Here's how the part is built. I have some questions about the finished solid (model axes, mm). Face numbers are marked on the shaded views. Give positions to 0.01 mm unless a question says otherwise; leave off trailing zeros. Loops run counter-clockwise (first coordinate to the right, second up) from the corner with the lowest first, then second, coordinate; pieces in that order, holes last. Notation, with made-up numbers: (17, -37.5) - (43, -37.5) arc R20 cw to (43, -18.5) - close; hole circle Ø9 at (-16, 36.25). An arc over 180 degrees is marked (long way). Use a Markdown table: item, result.
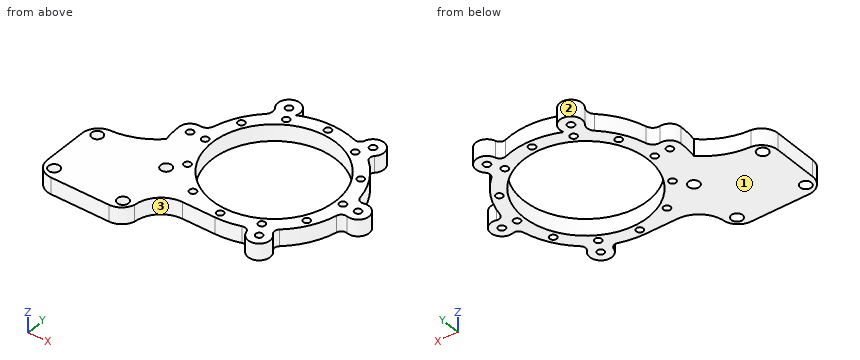
from build123d import *

# Parameters (mm, degrees)
SKETCH_2_R      = 1.25
SKETCH_2_R_2    = 22.5
SKETCH_2_R_3    = 2
EXTRUDE_1_DEPTH = 6
EXTRUDE_START   = -6
SKETCH_3_R      = 1.25
EXTRUDE_2_DEPTH = 6


with BuildPart() as part:
    # 草图2 → 凸台-拉伸1 (new body)
    with BuildSketch(Plane.XY):
        with BuildLine():
            ThreePointArc((11.071751856, 33.094337161), (3.155908846, 19.70243628), (-11.296671761, 13.946874314))
            ThreePointArc((-11.296671761, 13.946874314), (-15.015530454, 11.950947319), (-16.5, 8))
            Line((-16.5, 8), (-16.5, -8))
            ThreePointArc((-16.5, -8), (-14.742640687, -12.242640687), (-10.5, -14))
            Line((-10.5, -14), (10.5, -14))
            ThreePointArc((10.5, -14), (14.176185773, -12.741904487), (16.31070727, -9.495219388))
            ThreePointArc((16.31070727, -9.495219388), (19.407668924, -2.752662347), (26.297958971, 0))
            Line((26.297958971, 0), (37.996710384, 0))
            ThreePointArc((37.996710384, 0), (59.328544247, 44.855197033), (11.071751856, 33.094337161))
        make_face()
        with Locations((16.346075289, 15)):
            Circle(SKETCH_2_R, mode=Mode.SUBTRACT)
        with Locations((37.996710384, 2.5)):
            Circle(SKETCH_2_R, mode=Mode.SUBTRACT)
        with Locations((25.496710384, 5.849364905)):
            Circle(SKETCH_2_R, mode=Mode.SUBTRACT)
        with Locations((50.496710384, 5.849364905)):
            Circle(SKETCH_2_R, mode=Mode.SUBTRACT)
        with Locations((59.647345479, 15)):
            Circle(SKETCH_2_R, mode=Mode.SUBTRACT)
        with Locations((12.996710384, 27.5)):
            Circle(SKETCH_2_R, mode=Mode.SUBTRACT)
        with Locations((16.346075289, 40)):
            Circle(SKETCH_2_R, mode=Mode.SUBTRACT)
        with Locations((37.996710384, 27.5)):
            Circle(SKETCH_2_R_2, mode=Mode.SUBTRACT)
        with Locations((62.996710384, 27.5)):
            Circle(SKETCH_2_R, mode=Mode.SUBTRACT)
        with Locations((25.496710384, 49.150635095)):
            Circle(SKETCH_2_R, mode=Mode.SUBTRACT)
        with Locations((37.996710384, 52.5)):
            Circle(SKETCH_2_R, mode=Mode.SUBTRACT)
        with Locations((59.647345479, 40)):
            Circle(SKETCH_2_R, mode=Mode.SUBTRACT)
        with Locations((50.496710384, 49.150635095)):
            Circle(SKETCH_2_R, mode=Mode.SUBTRACT)
        with Locations((12.5, -10)):
            Circle(SKETCH_2_R_3, mode=Mode.SUBTRACT)
        with Locations((-12.5, 10)):
            Circle(SKETCH_2_R_3, mode=Mode.SUBTRACT)
        with Locations((12.5, 10)):
            Circle(SKETCH_2_R_3, mode=Mode.SUBTRACT)
        with Locations((-12.5, -10)):
            Circle(SKETCH_2_R_3, mode=Mode.SUBTRACT)
    extrude(amount=EXTRUDE_1_DEPTH)

    # 草图3 → 凸台-拉伸2 (add)
    # profile 1 of 5: a face of its own
    with BuildSketch(Plane.XY.offset(6).offset(EXTRUDE_START)):
        with BuildLine():
            ThreePointArc((67.447530056, 23.64004914), (72.496710384, 27.5), (67.447530056, 31.35995086))
            ThreePointArc((67.447530056, 31.35995086), (65.870885098, 31.588991044), (64.961839586, 32.897388914))
            ThreePointArc((64.961839586, 32.897388914), (65.496710384, 27.5), (64.961839586, 22.102611086))
            ThreePointArc((64.961839586, 22.102611086), (65.870885098, 23.411008956), (67.447530056, 23.64004914))
        make_face()
        with Locations((68.496710384, 27.5)):
            Circle(SKETCH_3_R, mode=Mode.SUBTRACT)
    # profile 2 of 5: a face of its own
    with BuildSketch(Plane.XY.offset(6).offset(EXTRUDE_START)):
        with BuildLine():
            ThreePointArc((56.064935722, 51.075182568), (55.246710384, 57.377876431), (49.379304718, 54.935133428))
            ThreePointArc((49.379304718, 54.935133428), (48.392627621, 53.684238934), (46.804999072, 53.551181363))
            ThreePointArc((46.804999072, 53.551181363), (51.746710384, 51.315698604), (56.153550899, 48.153792449))
            ThreePointArc((56.153550899, 48.153792449), (55.474967861, 49.59524789), (56.064935722, 51.075182568))
        make_face()
        with Locations((53.246710384, 53.913774815)):
            Circle(SKETCH_3_R, mode=Mode.SUBTRACT)
    # profile 3 of 5: a face of its own
    with BuildSketch(Plane.XY.offset(6).offset(EXTRUDE_START)):
        with BuildLine():
            ThreePointArc((49.379304718, 0.064866572), (55.246710384, -2.377876431), (56.064935722, 3.924817432))
            ThreePointArc((56.064935722, 3.924817432), (55.474967861, 5.40475211), (56.153550899, 6.846207551))
            ThreePointArc((56.153550899, 6.846207551), (51.746710384, 3.684301396), (46.804999072, 1.448818637))
            ThreePointArc((46.804999072, 1.448818637), (48.392627621, 1.315761066), (49.379304718, 0.064866572))
        make_face()
        with Locations((53.246710384, 1.086225185)):
            Circle(SKETCH_3_R, mode=Mode.SUBTRACT)
    # profile 4 of 5: a face of its own
    with BuildSketch(Plane.XY.offset(6).offset(EXTRUDE_START)):
        with BuildLine():
            ThreePointArc((26.477501839, 52.471140032), (22.209078662, 57.87747916), (19.535000313, 51.529468119))
            ThreePointArc((19.535000313, 51.529468119), (20.114268508, 49.473728128), (19.179054293, 47.553573727))
            ThreePointArc((19.179054293, 47.553573727), (22.630287457, 50.306206314), (26.477501839, 52.471140032))
        make_face()
        with Locations((22.746710384, 53.913774815)):
            Circle(SKETCH_3_R, mode=Mode.SUBTRACT)
    # profile 5 of 5: a face of its own
    with BuildSketch(Plane.XY.offset(6).offset(EXTRUDE_START)):
        with BuildLine():
            ThreePointArc((4.186169411, 20.637251344), (8.570590949, 26.345313518), (11.071751856, 33.094337161))
            ThreePointArc((11.071751856, 33.094337161), (11.144241114, 33.432528477), (11.220978054, 33.769781351))
            ThreePointArc((11.220978054, 33.769781351), (10.025683209, 31.99978526), (7.955726823, 31.473575708))
            ThreePointArc((7.955726823, 31.473575708), (4.835513826, 30.486307566), (3.496710384, 27.5))
            ThreePointArc((3.496710384, 27.5), (3.669507879, 24.051352697), (4.186169411, 20.637251344))
        make_face()
        with Locations((7.496710384, 27.5)):
            Circle(SKETCH_3_R, mode=Mode.SUBTRACT)
    extrude(amount=EXTRUDE_2_DEPTH)


solid = part.part
(1) Suppose I cut it at A-A on y = 35. Write out the boundary of the cut face in (x, z), plus the area to 3 significant figures.
A:
| item | result |
|---|---|
| outline | (11.54, 0) - (16.78, 0) - (16.78, 6) - (11.54, 6) - close; (59.21, 0) - (64.45, 0) - (64.45, 6) - (59.21, 6) - close |
| area | 62.9 mm2 |
(2) If I drill on line 1 (X direction, y = 16, z = 3.15); line 2 (Y direction, x = 56.5, z = 3.15); line 3 (X direction, y = -8.5, z = 3.2), over which ranges is the centre line in solid material (lowest first)?
A:
| item | result |
|---|---|
| line 1 | -2.7 to 15.6, 17.1 to 18.66, 57.34 to 58.9, 60.4 to 62.98 |
| line 2 | -1.24 to 3.41, 7.16 to 14.7, 40.3 to 47.84, 51.59 to 56.24 |
| line 3 | -16.48 to -13.82, -11.18 to 11.18, 13.82 to 16.41 |
(3) We'd pull the mould along Y, two halves only. Please class the marked faces 1, 2 and 3: pulls with the +Y half, pulls with the -Y half, needs draft (parallel to the pull), parting line crosses it, or undercut.
A:
| item | result |
|---|---|
| face 1 | needs draft |
| face 2 | undercut |
| face 3 | pulls with the -Y half |
(4) Suppose I cut it at B-B on x = 43. Write out the boundary of the cut face in (y, z).
A:
| item | result |
|---|---|
| outline | (0.46, 0) - (5.56, 0) - (5.56, 6) - (0.46, 6) - close; (49.44, 0) - (54.54, 0) - (54.54, 6) - (49.44, 6) - close |
(5) Suppose I cut it at D-D on z = 3.3. Count the separate pieces of the cut face and the enclosed holes in it, plus the area to 3 significant figures.
A:
| item | result |
|---|---|
| separate pieces | 1 |
| enclosed holes | 22 |
| area | 2,000 mm2 |
(6) Will these pins go through, and if not, where does the flat tip stop? pin 1 (2 mm diameter, centred on y = 42.5, z = 4, fed in from +X); pin 2 (3 mm diameter, centred on y = 14.5, z = 1.5, fed in from -X); pin 3 (1.5 mm diameter, centred on x = 40, z = 1.5, fed in from -Y).
A:
| item | result |
|---|---|
| pin 1 | x = 61.67 |
| pin 2 | x = -13.82 |
| pin 3 | y = 0.03 |
(7) Suppose I cut it at C-C on x = -12.5. Write out the boundary of the cut face in (y, z), plus the area to 3 significant figures.
A:
| item | result |
|---|---|
| outline | (-13.66, 0) - (-12, 0) - (-12, 6) - (-13.66, 6) - close; (-8, 0) - (8, 0) - (8, 6) - (-8, 6) - close; (12, 0) - (13.66, 0) - (13.66, 6) - (12, 6) - close |
| area | 116 mm2 |
